The listing builds one solid part. Answer for the finished solid, in the listing's coordinates (mm). A direction names the side the tool comes from. Coordinates: 2 decimals unless noted, no trailing zeros. Write each loop counter-clockwise with the first axis right and the second up, starting at its lowest first coordinate (ties: lowest second). Pieces come first, ordered by that corner, then holes.
from build123d import *

# Parameters (mm, degrees)
SKETCH2_W               = 80
SKETCH2_H               = 47.65
BOSS_EXTRUDE1_DEPTH     = 3.175
SKETCH3_W               = 15
SKETCH3_H               = 3.5
BOSS_EXTRUDE2_DEPTH     = 3.175
SKETCH4_W               = 3.5
SKETCH4_H               = 15
BOSS_EXTRUDE3_DEPTH     = 3.175
MIRROR2_COPY_1_SKETCH_W = 3.5
MIRROR2_COPY_1_SKETCH_H = 15
MIRROR2_COPY_1_DEPTH    = 3.175
MIRROR2_COPY_2_SKETCH_W = 3.5
MIRROR2_COPY_2_SKETCH_H = 15
MIRROR2_COPY_2_DEPTH    = 3.175
CUT_EXTRUDE1_DEPTH      = 10
MIRROR4_COPY_1_DEPTH    = 10
CUT_EXTRUDE2_DEPTH      = 10
LPATTERN1_COUNT         = 3
LPATTERN1_PITCH         = 5
MIRROR5_COPY_1_DEPTH    = 10
MIRROR5_COPY_2_DEPTH    = 10
CUT_EXTRUDE6_DEPTH      = 52.468303353
CUT_EXTRUDE6_DEPTH_BACK = 52.468303353
SKETCH7_R               = 1.55


with BuildPart() as part:
    # Sketch2 → Boss-Extrude1 (new body)
    with BuildSketch(Plane(origin=(0, 0, 0), x_dir=(1, 0, 0), z_dir=(0, 1, 0))):
        Rectangle(SKETCH2_W, SKETCH2_H)
    extrude(amount=BOSS_EXTRUDE1_DEPTH)

    # Sketch3 → Boss-Extrude2 (add)
    with BuildSketch(Plane(origin=(0, 3.175, 0), x_dir=(1, 0, 0), z_dir=(0, 1, 0))):
        with Locations((0, 25.575)):
            Rectangle(SKETCH3_W, SKETCH3_H)
    boss_extrude2 = extrude(amount=-BOSS_EXTRUDE2_DEPTH)

    # Sketch4 → Boss-Extrude3 (add)
    with BuildSketch(Plane(origin=(0, 3.175, 0), x_dir=(1, 0, 0), z_dir=(0, 1, 0))):
        with Locations((-41.75, 0)):
            Rectangle(SKETCH4_W, SKETCH4_H)
    boss_extrude3 = extrude(amount=-BOSS_EXTRUDE3_DEPTH)

    # Mirror1: Boss-Extrude3 across plane
    add(boss_extrude3.mirror(Plane(origin=(0, 0, 0), x_dir=(0, 0, 1), z_dir=(1, 0, 0))))

    # Mirror2: Boss-Extrude2 across plane
    add(boss_extrude2.mirror(Plane.XY))

    # Mirror2 copy 1 sketch → Mirror2 copy 1 (add)
    with BuildSketch(Plane(origin=(0, 3.175, 0), x_dir=(-1, 0, 0), z_dir=(0, 1, 0))):
        with Locations((-41.75, 0)):
            Rectangle(MIRROR2_COPY_1_SKETCH_W, MIRROR2_COPY_1_SKETCH_H)
    extrude(amount=-MIRROR2_COPY_1_DEPTH)

    # Mirror2 copy 2 sketch → Mirror2 copy 2 (add)
    with BuildSketch(Plane(origin=(0, 3.175, 0), x_dir=(1, 0, 0), z_dir=(0, 1, 0))):
        with Locations((-41.75, 0)):
            Rectangle(MIRROR2_COPY_2_SKETCH_W, MIRROR2_COPY_2_SKETCH_H)
    extrude(amount=-MIRROR2_COPY_2_DEPTH)

    # Sketch5 → Cut-Extrude1 (cut)
    with BuildSketch(Plane(origin=(0, 3.175, 0), x_dir=(1, 0, 0), z_dir=(0, 1, 0))):
        Polygon((-40, 13.55), (-36, 13.55), (-36, 14.55), (-32.5, 14.55), (-32.5, 10.45), (-36, 10.45), (-36, 11.45), (-40, 11.45), align=None)
    cut_extrude1 = extrude(amount=-CUT_EXTRUDE1_DEPTH, mode=Mode.SUBTRACT)

    # Mirror3: Cut-Extrude1 across plane
    add(cut_extrude1.mirror(Plane.XY), mode=Mode.SUBTRACT)

    # Mirror4: Cut-Extrude1 across plane
    add(cut_extrude1.mirror(Plane(origin=(0, 0, 0), x_dir=(0, 0, 1), z_dir=(1, 0, 0))), mode=Mode.SUBTRACT)

    # Mirror4 copy 1 sketch → Mirror4 copy 1 (cut)
    with BuildSketch(Plane(origin=(0, 3.175, 0), x_dir=(-1, 0, 0), z_dir=(0, 1, 0))):
        Polygon((-40, 13.55), (-36, 13.55), (-36, 14.55), (-32.5, 14.55), (-32.5, 10.45), (-36, 10.45), (-36, 11.45), (-40, 11.45), align=None)
    extrude(amount=-MIRROR4_COPY_1_DEPTH, mode=Mode.SUBTRACT)

    # Sketch6 → Cut-Extrude2 (cut)
    with BuildSketch(Plane(origin=(0, 3.175, 0), x_dir=(1, 0, 0), z_dir=(0, 1, 0))):
        with BuildLine():
            Line((5.15, -9), (5.15, 9))
            ThreePointArc((5.15, 9), (6.5, 10.35), (7.85, 9))
            Line((7.85, 9), (7.85, -9))
            ThreePointArc((7.85, -9), (6.5, -10.35), (5.15, -9))
        make_face()
    cut_extrude2 = extrude(amount=-CUT_EXTRUDE2_DEPTH, mode=Mode.SUBTRACT)

    # LPattern1: Cut-Extrude2 ×3
    with Locations(*[(i * LPATTERN1_PITCH, 0, 0) for i in range(1, LPATTERN1_COUNT)]):
        add(cut_extrude2, mode=Mode.SUBTRACT)

    # Mirror5: Cut-Extrude2 across plane
    add(cut_extrude2.mirror(Plane(origin=(0, 0, 0), x_dir=(0, 0, 1), z_dir=(1, 0, 0))), mode=Mode.SUBTRACT)

    # Mirror5 copy 1 sketch → Mirror5 copy 1 (cut)
    with BuildSketch(Plane(origin=(-5, 3.175, 0), x_dir=(-1, 0, 0), z_dir=(0, 1, 0))):
        with BuildLine():
            Line((5.15, 9), (5.15, -9))
            ThreePointArc((5.15, -9), (6.5, -10.35), (7.85, -9))
            Line((7.85, -9), (7.85, 9))
            ThreePointArc((7.85, 9), (6.5, 10.35), (5.15, 9))
        make_face()
    extrude(amount=-MIRROR5_COPY_1_DEPTH, mode=Mode.SUBTRACT)

    # Mirror5 copy 2 sketch → Mirror5 copy 2 (cut)
    with BuildSketch(Plane(origin=(-10, 3.175, 0), x_dir=(-1, 0, 0), z_dir=(0, 1, 0))):
        with BuildLine():
            Line((5.15, 9), (5.15, -9))
            ThreePointArc((5.15, -9), (6.5, -10.35), (7.85, -9))
            Line((7.85, -9), (7.85, 9))
            ThreePointArc((7.85, 9), (6.5, 10.35), (5.15, 9))
        make_face()
    extrude(amount=-MIRROR5_COPY_2_DEPTH, mode=Mode.SUBTRACT)

    # Sketch7 → Cut-Extrude6 (cut, two sides: drawn at the far end of the back side and taken through both)
    with BuildSketch(Plane(origin=(0, 0, 0), x_dir=(1, 0, 0), z_dir=(0, 1, 0)).offset(-CUT_EXTRUDE6_DEPTH_BACK)):
        with Locations(Location((0, 0, 0), (0, 0, 270))):
            Circle(SKETCH7_R)
    extrude(amount=CUT_EXTRUDE6_DEPTH + CUT_EXTRUDE6_DEPTH_BACK, mode=Mode.SUBTRACT)


solid = part.part
1. A tool of negligible diameter and unlimited length cuts with its end or side. For faces 4 (the flat face through (0, 2, -27.325)), 5 (the flat face through (24, 2, 23.825)), 6 (the cylindrical face through (-6.53, 1.61, 10.35)), 7 (the flat face through (42, 2, -7.5)), 8 (the flat face through (-24, 2, 23.825)), from which of +Z, -Z, +X, -X, +Y, -Y can it reach the whole face along a straight path? Write none if from no direction.
Results found:
face 4: -Z, +X, -X, +Y, -Y
face 5: +Z, +X, +Y, -Y
face 6: +Y, -Y
face 7: -Z, +X, +Y, -Y
face 8: +Z, -X, +Y, -Y
2. For a pull along X with two mould halves and no side action, classify faces 1 (the flat face through (-42, 2, -7.5)), 2 (the flat face through (40, 2, 19)), 3 (the cylindrical face through (16.53, 1.61, 10.35)) as pulls with the +X half, pulls with the -X half, needs draft (parallel to the pull), parting line crosses it, or undercut.
Results found:
face 1: needs draft
face 2: pulls with the +X half
face 3: undercut
3. Find the intervals of material crossed by L1, parallel to Z at x = -38.5, y = 1.4 (3 decimals); L2, parallel to Z at x = 0, y = 2.35 (3 decimals); L3, parallel to Z at x = 6.5, y = 1.55 (3 decimals), in increasing order.
Results found:
L1: z = -23.825 to -13.55, -11.45 to 11.45, 13.55 to 23.825
L2: z = -27.325 to -1.55, 1.55 to 27.325
L3: z = -27.325 to -10.35, 10.35 to 27.325
4. Section B-B on x = 0 is taken. Give the vertices of the cut face in (y, z) (3 decimals).
Results found:
outline: (0, -27.325) - (3.175, -27.325) - (3.175, -1.55) - (0, -1.55) - close; (0, 1.55) - (3.175, 1.55) - (3.175, 27.325) - (0, 27.325) - close
5. Section D-D on x = 11.5 is taken. Give the vertices of the cut face in (y, z) (3 decimals), then the cut area to 3 significant figures.
Results found:
outline: (0, -23.825) - (3.175, -23.825) - (3.175, -10.35) - (0, -10.35) - close; (0, 10.35) - (3.175, 10.35) - (3.175, 23.825) - (0, 23.825) - close
area: 85.6 mm2
6. Section A-A on z = 0 is taken. State how many separate pieces and enclosed holes the cut face has, then the cut area to 3 significant figures.
Results found:
separate pieces: 8
enclosed holes: 0
area: 215 mm2
7. Flat-ended cylindrical pins translate along their axes: P1, Ø1, axis at y = 1, z = -16.5, coming from the +X side; P2, Ø1, axis at x = -34.5, y = 1.5, coming from the -Z side (3 decimals); P3, Ø1.6, axis at x = -41.5, y = 1.5, coming from the -Z side. Find the tip coordinate at first contact, or state that the pin passes through.
Results found:
P1: stops at x = 40
P2: stops at z = -23.825
P3: stops at z = -7.5
8. Section C-C on z = 6 is taken. Give the vertices of the cut face in (x, y) (3 decimals).
Results found:
outline: (-43.5, 0) - (-17.85, 0) - (-17.85, 3.175) - (-43.5, 3.175) - close; (-15.15, 0) - (-12.85, 0) - (-12.85, 3.175) - (-15.15, 3.175) - close; (-10.15, 0) - (-7.85, 0) - (-7.85, 3.175) - (-10.15, 3.175) - close; (-5.15, 0) - (5.15, 0) - (5.15, 3.175) - (-5.15, 3.175) - close; (7.85, 0) - (10.15, 0) - (10.15, 3.175) - (7.85, 3.175) - close; (12.85, 0) - (15.15, 0) - (15.15, 3.175) - (12.85, 3.175) - close; (17.85, 0) - (43.5, 0) - (43.5, 3.175) - (17.85, 3.175) - close
